Geometry: final body of the model. Coordinates: model frame, mm. A direction names the side the tool comes from. Give positions to 0.01 mm unless a question says otherwise; leave off trailing zeros. Order: outer loops, then holes, each group sorted by start corner. A loop starts at its lowest first (then second) coordinate and runs counter-clockwise, first axis right, second up. Notation, with made-up numbers: (40, 77) - (48, 77) arc R19 ccw to (48, 95) - close; hole circle Ø3 at (5, -18). An arc over 180 degrees is marked (long way). One line per question, with ' | ' between items. Start each with the question number.
Autodesk Inventor part; units mm, degrees
ref_plane "YZ Plane" through (0, 0, 0) normal (1, 0, 0) x (0, 1, 0)
ref_plane "XZ Plane" through (0, 0, 0) normal (0, 1, 0) x (-1, 0, 0)
ref_plane "XY Plane" through (0, 0, 0) normal (0, 0, 1) x (1, 0, 0)
sketch "Sketch1" plane through (0, 0, 0) normal (0, 1, 0) x (-1, 0, 0)
  circle A0 centre (0, 0) radius 2.875
  dimension "d0" = 5.75
extrude "Extrusion1" add sketch "Sketch1" along normal mid plane 6.75
sketch "Sketch2" plane through (0, -3.375, 0) normal (0, -1, 0) x (1, 0, 0)
  circle A0 centre (0, 0) radius 2
  dimension "d3" = 4
extrude "Extrusion2" add sketch "Sketch2" along normal blind 0.75
sketch "Sketch3" plane through (0, 3.375, 0) normal (0, 1, 0) x (1, 0, 0)
  circle A0 centre (0, 0) radius 5
  dimension "d6" = 10
extrude "Extrusion3" add sketch "Sketch3" along normal blind 1.5
sketch "Sketch5" plane through (0, 0, 0) normal (0, 0, 1) x (1, 0, 0)
  line L0 (5, 4.875) -> (-5, 4.875)
  line L1 (0, 4.875) -> (0, 7.225)
  line L2 (0, 4.875) -> (5, 4.875)
  arc A0 (5, 4.875) -> (0, 7.225) centre (-0.0027, 0.725) ccw
  line L3 (0, 4.875) -> (0, 12.9944) construction
  point P0 (0, 0)
  dimension "d9" = 2.35
  dimension "d10" = 6.5
revolve "Revolution1" add sketch "Sketch5" angle 360 about axis through (0, 4.875, 0) along (0, 1, 0)
sketch "Sketch6" plane through (0, 0, 0) normal (0, 0, 1) x (1, 0, 0)
  line L0 (5, 4.875) -> (-5, 4.875)
  line L1 (0, 5.755) -> (0.75, 5.755)
  line L2 (0.75, 5.755) -> (0.75, 8.519)
  line L3 (0.75, 8.519) -> (-0.75, 8.519)
  line L4 (-0.75, 8.519) -> (-0.75, 5.755)
  line L5 (-0.75, 5.755) -> (0, 5.755)
  point P0 (0, 0)
  dimension "d13" = 0.75
  dimension "d14" = 1.5
extrude "Extrusion4" cut sketch "Sketch6" against normal mid plane 15
properties part number "Pieza 1 KAS" material "Steel, Galvanized"
(1) Access query for faces 4 (the flat face through (-0.75, 6, 0)), 5 (the cylindrical face through (-1.08, 4.11, -4.88)), 6 (the flat face through (2, -3.375, -1)). Directions: +Z, -Z, +X, -X, +Y, -Y. A direction counts if a zero-diameter tool reaches every point of the face in a straight line with its end or side. Return the directions, or none.
(2) Pull-direction query (X, two-part tool) for faces 1 (the cylindrical face through (0.37, 0.05, 2.85)), 2 (the flat face through (0.75, 6, 0)), 3 (the flat face through (0, -4.125, 0)); classes: +X half, -X half, draft (parallel to the pull), parting line (faces both ways), or undercut.
(3) Material intervals for line 1 along Y through (x, z) = (0, -2.25) (3 decimals); line 2 along Y through (x, z) = (0.5, -4) (3 decimals); line 3 along Z through (x, y) = (-1.25, -0.25), sorted ascending. Write a range as from..to.
(4) Contact query for flat-ended pins moving along their axis: P1, Ø0.8, axis at x = 0, z = -0.5, coming from the +Y side (3 decimals); P2, Ø1.6, axis at y = 6.5, z = 0, coming from the -X side; P3, Ø3, axis at x = 0.5, y = -0.5, coming from the +Z side (3 decimals). Output: stop coordinate, or through.
(5) Cut plane A-A, the plane y = 3. Return the cut outline in (x, z) (3 decimals), plus the area to 3 significant figures.
Results are:
1) face 4: +Z, -Z, +Y | face 5: +Y, -Y | face 6: -Y
2) face 1: parting line | face 2: undercut | face 3: draft
3) line 1: -3.375..5.755 | line 2: 3.375..5.755 | line 3: -2.59..2.59
4) P1: y = 5.755 | P2: x = -4.18 | P3: z = 2.875
5) outline: circle Ø5.75 at (0, 0) | area: 26.0 mm2
